Source: CAD feature listing. Evaluate the final solid. Frame: model axes, mm. A direction names the side the tool comes from. Coordinates: 2 decimals unless noted, no trailing zeros. Order: outer loops, then holes, each group sorted by start corner. A loop starts at its lowest first (then second) coordinate and runs counter-clockwise, first axis right, second up.
Solid Edge part; units mm, degrees
sketch "Sketch1" plane through (0, 0, 0) normal (0, -1, 0) x (1, 0, 0)
  circle A0 centre (0, 0) radius 2
extrude "Protrusion1" add sketch "Sketch1" along normal blind 6.7
sketch "Sketch2" plane through (0, 0, 0) normal (0, 1, 0) x (1, 0, 0)
  line L0 (2.4942, -1.4332) -> (0, -2.8732)
  line L1 (-2.4942, -1.4332) -> (0, -2.8732)
  line L2 (-2.4942, 1.4468) -> (-2.4942, -1.4332)
  line L3 (0, 2.8868) -> (-2.4942, 1.4468)
  line L4 (0, 2.8868) -> (2.4942, 1.4468)
  line L5 (2.4942, 1.4468) -> (2.4942, -1.4332)
extrude "ExtrudedProtrusion_2" add sketch "Sketch2" along normal blind 2
fillet "Round_1" radius 0.2 12 edges at (1.2471, 0, 2.1532) (-1.2471, 0, 2.1532) (2.4942, 0, -0.0068) (1.2471, 0, -2.1668) (-1.2471, 0, -2.1668) (-2.4942, 0, -0.0068) (1.2471, 2, 2.1532) (-1.2471, 2, 2.1532) (-2.4942, 2, -0.0068) (-1.2471, 2, -2.1668) (1.2471, 2, -2.1668) (2.4942, 2, -0.0068)
fillet "Round_2" radius 0.2 18 edges at (0, 1, 2.8732) (0, 0.0586, 2.8056) (0, 1.9414, 2.8056) (2.4942, 1, 1.4332) (2.4356, 0.0586, 1.3994) (2.4356, 1.9414, 1.3994) (2.4942, 1, -1.4468) (2.4356, 0.0586, -1.4129) (2.4356, 1.9414, -1.4129) (-2.4942, 1, 1.4332) (-2.4356, 0.0586, 1.3994) (-2.4356, 1.9414, 1.3994) (0, 1, -2.8868) (0, 0.0586, -2.8191) (0, 1.9414, -2.8191) (-2.4942, 1, -1.4468) (-2.4356, 0.0586, -1.4129) (-2.4356, 1.9414, -1.4129)
chamfer "Chamfer_1" distance 0.5 angle 45 1 edges at (-2, -6.7, 0)
properties material "PVC"
1. Access query for faces 1 (the face through (-1.203, 0.06, 2.113)), 2 (the face through (-2, 0, -1)). Directions: +Z, -Z, +X, -X, +Y, -Y. A direction counts if a zero-diameter tool reaches every point of the face in a straight line with its end or side. Return the directions, or none.
Findings:
face 1: +Z, -X, -Y
face 2: -Y
2. Section query A-A on y = 1. Return loops of the section in (x, z).
Findings:
outline: (-2.49, -1.33) arc R0.2 ccw to (-2.39, -1.5) - (-0.1, -2.83) arc R0.2 ccw to (0.1, -2.83) - (2.39, -1.5) arc R0.2 ccw to (2.49, -1.33) - (2.49, 1.32) arc R0.2 ccw to (2.39, 1.49) - (0.1, 2.82) arc R0.2 ccw to (-0.1, 2.82) - (-2.39, 1.49) arc R0.2 ccw to (-2.49, 1.32) - close
3. Pin query (flat end, axial travel): P1, Ø1, axis at x = 1, y = -5.5, coming from the -Z side. Return the tip coordinate at first contact, or that it passes through.
Findings:
P1: stops at z = -1.94
4. Section query B-B on z = 0. Return loops of the section in (x, y), plus the area to 3 significant figures.
Findings:
outline: (-2.49, 0.2) arc R0.2 ccw to (-2.29, 0) - (-2, 0) - (-2, -6.2) - (-1.5, -6.7) - (1.5, -6.7) - (2, -6.2) - (2, 0) - (2.29, 0) arc R0.2 ccw to (2.49, 0.2) - (2.49, 1.8) arc R0.2 ccw to (2.29, 2) - (-2.29, 2) arc R0.2 ccw to (-2.49, 1.8) - close
area: 36.5 mm2
5. Ray query, line 1 (Y direction, x = 2.3, z = 0.95); line 2 (X direction, y = -5.75, z = -0.8); line 3 (Y direction, x = 1, z = -2.25). Return the intervals inside material, ascending.
Findings:
line 1: y = 0 to 2
line 2: x = -1.83 to 1.83
line 3: y = 0.07 to 1.93
